```python
from build123d import *

# Parameters (mm, degrees)
EXTRUDE_1_DEPTH        = 3
SHEET_START            = -1
SHEET_METAL_1_DEPTH    = 1
SM_EDGE_FLANGE_1_DEPTH = 60
CUT_EXTRUDE_1_DEPTH    = 149.811702088
CUT_EXTRUDE_2_DEPTH    = 114.368696469
CUT_EXTRUDE_4_DEPTH    = 114.368696469
MIRROR_6_COPY_1_DEPTH  = 149.811702088
SKETCH_13_R            = 5.1
CUT_EXTRUDE_5_DEPTH    = 155.10011472
FILLET_1_R             = 10
CUT_EXTRUDE_6_REACH    = 110.409
SKETCH_15_R            = 2.1


# Read off the part's stored shape, not the designer's step: 轉換-實體1
# Sheet-metal steps are written as plain solids
with BuildPart() as part:
    # Sketch 1 → 填料-伸長1 (new body)
    with BuildSketch(Plane(origin=(0, 0, 0), x_dir=(1, 0, 0), z_dir=(0, 1, 0))):
        Polygon((30, 51.961524227), (-30, 51.961524227), (-60, 0), (-30, -51.961524227), (30, -51.961524227), (60, 0), align=None)
    extrude(amount=EXTRUDE_1_DEPTH)

    # Sheet Metal 1 outline → Sheet Metal 1 (add)
    with BuildSketch(Plane(origin=(0, 0, 0), x_dir=(1, 0, 0), z_dir=(0, 1, 0)).offset(SHEET_START)):
        Polygon((-30, 51.961524227), (-60, 0), (-30, -51.961524227), (30, -51.961524227), (60, 0), (30, 51.961524227), align=None)
    extrude(amount=SHEET_METAL_1_DEPTH)

    # 邊線-凸緣1 section (across the edge) → 邊線-凸緣1 (add)
    with BuildSketch(Plane(origin=(-30, 3, 54.961524227), x_dir=(0, 0, -1), z_dir=(1, 0, 0))):
        with BuildLine():
            Line((-4, 1), (-4, 76))
            Line((-4, 76), (0, 76))
            Line((0, 76), (0, 1))
            ThreePointArc((0, 1), (0.292893219, 0.292893219), (1, 0))
            Line((1, 0), (3, 0))
            Line((3, 0), (3, -4))
            Line((3, -4), (1, -4))
            ThreePointArc((1, -4), (-2.535533906, -2.535533906), (-4, 1))
        make_face()
    sm_edge_flange_1 = extrude(amount=SM_EDGE_FLANGE_1_DEPTH)

    # 草圖9 → 除料-伸長1 (cut, symmetric)
    with BuildSketch(Plane.XY.offset(58.961524227)):
        Polygon((-30, 79), (-30, 14), (-10, 79), align=None)
    cut_extrude_1 = extrude(amount=CUT_EXTRUDE_1_DEPTH, both=True, mode=Mode.SUBTRACT)

    # 草圖10 → 除料-伸長2 (cut, through all)
    with BuildSketch(Plane(origin=(0, 3, 0), x_dir=(1, 0, 0), z_dir=(0, 1, 0))):
        Polygon((10, 17.320508076), (-10, 17.320508076), (-20, 0), (-10, -17.320508076), (10, -17.320508076), (20, 0), align=None)
    extrude(amount=-CUT_EXTRUDE_2_DEPTH, mode=Mode.SUBTRACT)

    # 草圖12 → 除料-伸長4 (cut, symmetric)
    with BuildSketch(Plane(origin=(0, 3, 0), x_dir=(1, 0, 0), z_dir=(0, 1, 0))):
        Polygon((50, 295.043861202), (50, 17.320508076), (50, -17.320508076), (50, -295.043861202), (605.446706252, -295.043861202), (605.446706252, 295.043861202), align=None)
    cut_extrude_4 = extrude(amount=CUT_EXTRUDE_4_DEPTH, both=True, mode=Mode.SUBTRACT)

    # 鏡射1: 除料-伸長1 across plane
    add(cut_extrude_1.mirror(Plane(origin=(0, 0, 0), x_dir=(0, 0, 1), z_dir=(1, 0, 0))), mode=Mode.SUBTRACT)

    # 鏡射6: 邊線-凸緣1, 除料-伸長1 across plane
    add(sm_edge_flange_1.mirror(Plane.XY))
    add(cut_extrude_1.mirror(Plane.XY), mode=Mode.SUBTRACT)

    # 鏡射6 copy 1 sketch → 鏡射6 copy 1 (cut, symmetric)
    with BuildSketch(Plane(origin=(0, 0, -58.961524227), x_dir=(-1, 0, 0), z_dir=(0, 0, -1))):
        Polygon((-30, 79), (-30, 14), (-10, 79), align=None)
    extrude(amount=MIRROR_6_COPY_1_DEPTH, both=True, mode=Mode.SUBTRACT)

    # 草圖13 → 除料-伸長5 (cut, through all)
    with BuildSketch(Plane.XY.offset(58.961524227)):
        with Locations((0, 60)):
            Circle(SKETCH_13_R)
    extrude(amount=-CUT_EXTRUDE_5_DEPTH, mode=Mode.SUBTRACT)

    # 圓角1
    fillet_1_edges = [part.edges().sort_by_distance(p)[0] for p in [
        (10, 79, 56.961524227),
        (10, 79, -56.961524227),
        (-10, 79, -56.961524227),
        (-10, 79, 56.961524227),
    ]]
    fillet(fillet_1_edges, radius=FILLET_1_R)

    # 鏡射7: 除料-伸長4 across plane
    add(cut_extrude_4.mirror(Plane(origin=(0, 0, 0), x_dir=(0, 0, 1), z_dir=(1, 0, 0))), mode=Mode.SUBTRACT)

    # 草圖15 → 除料-伸長6 (cut, up to next)
    with BuildSketch(Plane(origin=(0, 3, 0), x_dir=(1, 0, 0), z_dir=(0, 1, 0)), mode=Mode.PRIVATE) as cut_extrude_6_sk1:
        with Locations(Location((-35, 0, 0), (0, 0, 270))):
            Circle(SKETCH_15_R)
    cut_extrude_6_tool1 = extrude(cut_extrude_6_sk1.sketch, amount=-CUT_EXTRUDE_6_REACH, mode=Mode.PRIVATE) & part.part
    # 草圖15 → 除料-伸長6 (cut, up to next)
    with BuildSketch(Plane(origin=(0, 3, 0), x_dir=(1, 0, 0), z_dir=(0, 1, 0)), mode=Mode.PRIVATE) as cut_extrude_6_sk2:
        with Locations(Location((-25, 35, 0), (0, 0, 270))):
            Circle(SKETCH_15_R)
    cut_extrude_6_tool2 = extrude(cut_extrude_6_sk2.sketch, amount=-CUT_EXTRUDE_6_REACH, mode=Mode.PRIVATE) & part.part
    # 草圖15 → 除料-伸長6 (cut, up to next)
    with BuildSketch(Plane(origin=(0, 3, 0), x_dir=(1, 0, 0), z_dir=(0, 1, 0)), mode=Mode.PRIVATE) as cut_extrude_6_sk3:
        with Locations(Location((25, 35, 0), (0, 0, 270))):
            Circle(SKETCH_15_R)
    cut_extrude_6_tool3 = extrude(cut_extrude_6_sk3.sketch, amount=-CUT_EXTRUDE_6_REACH, mode=Mode.PRIVATE) & part.part
    # 草圖15 → 除料-伸長6 (cut, up to next)
    with BuildSketch(Plane(origin=(0, 3, 0), x_dir=(1, 0, 0), z_dir=(0, 1, 0)), mode=Mode.PRIVATE) as cut_extrude_6_sk4:
        with Locations(Location((25, -35, 0), (0, 0, 270))):
            Circle(SKETCH_15_R)
    cut_extrude_6_tool4 = extrude(cut_extrude_6_sk4.sketch, amount=-CUT_EXTRUDE_6_REACH, mode=Mode.PRIVATE) & part.part
    # 草圖15 → 除料-伸長6 (cut, up to next)
    with BuildSketch(Plane(origin=(0, 3, 0), x_dir=(1, 0, 0), z_dir=(0, 1, 0)), mode=Mode.PRIVATE) as cut_extrude_6_sk5:
        with Locations(Location((-25, -35, 0), (0, 0, 270))):
            Circle(SKETCH_15_R)
    cut_extrude_6_tool5 = extrude(cut_extrude_6_sk5.sketch, amount=-CUT_EXTRUDE_6_REACH, mode=Mode.PRIVATE) & part.part
    # 草圖15 → 除料-伸長6 (cut, up to next)
    with BuildSketch(Plane(origin=(0, 3, 0), x_dir=(1, 0, 0), z_dir=(0, 1, 0)), mode=Mode.PRIVATE) as cut_extrude_6_sk6:
        with Locations(Location((35, 0, 0), (0, 0, 270))):
            Circle(SKETCH_15_R)
    cut_extrude_6_tool6 = extrude(cut_extrude_6_sk6.sketch, amount=-CUT_EXTRUDE_6_REACH, mode=Mode.PRIVATE) & part.part
    add(cut_extrude_6_tool1.solids().sort_by_distance((-35, 3, 0))[0], mode=Mode.SUBTRACT)
    add(cut_extrude_6_tool2.solids().sort_by_distance((-25, 3, -35))[0], mode=Mode.SUBTRACT)
    add(cut_extrude_6_tool3.solids().sort_by_distance((25, 3, -35))[0], mode=Mode.SUBTRACT)
    add(cut_extrude_6_tool4.solids().sort_by_distance((25, 3, 35))[0], mode=Mode.SUBTRACT)
    add(cut_extrude_6_tool5.solids().sort_by_distance((-25, 3, 35))[0], mode=Mode.SUBTRACT)
    add(cut_extrude_6_tool6.solids().sort_by_distance((35, 3, 0))[0], mode=Mode.SUBTRACT)


solid = part.part
```
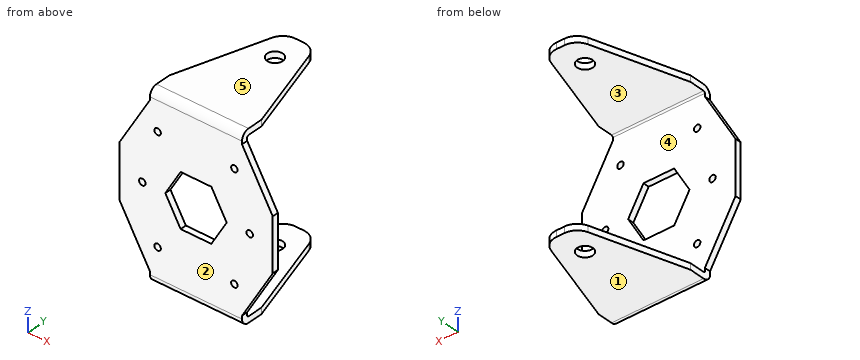
Part model, mm, in its own coordinate system. Face numbers are marked on the shaded views. A direction names the side the tool comes from. Round coordinates to 2 decimals unless told otherwise and drop trailing zeros. Write each loop counter-clockwise with the first axis right and the second up, starting at its lowest first coordinate (ties: lowest second). Pieces come first, ordered by that corner, then holes. Notation, with made-up numbers: M -14,71.25 L 40,71.25 A24 cw 40,85.25 Z; hole C 46,17.5 d2. An arc over 180 degrees is marked long. Answer as CSV lines item,"result". Start each with the question number.
1) Band-saw the part on B-B (y = 47). List the corners of the cut face in (x, z), then the cut area to 3 significant figures.
2) Drill centre lines: L1, parallel to X at y = 1, z = 0; L2, parallel to Z at x = -19.5, y = 38; L3, parallel to Y at x = 22.5, z = 49. Where is each one in solid material? Low to high.
3) Band-saw the part on A-A (x = 25). List the corners of the cut face in (y, z).
4) Which spindle directions (+Z, -Z, +X, -X, +Y, -Y) get a long thin tool onto all of the face, cutting with end or side? Do the marked faces 4 and 5. Say none if no direction does.
5) Band-saw the part on C-C (z = 35). List the corners of the cut face in (x, y), then the cut area to 3 significant figures.
6) Band-saw the part on D-D (x = 14). List the corners of the cut face in (y, z), then the cut area to 3 significant figures.
7) Drop flat-ended pins along their axis: pin 1 (2 mm diameter, centred on x = 4.5, y = 0.5, fed in from +Z); pin 2 (5.5 mm diameter, centred on y = 7, z = 56, fed in from +X); pin 3 (5.5 mm diameter, centred on x = -25, z = 35, fed in from +Y). Give the stop position or say it passes through.
8) Mould opens along Z. For the marked faces 1, 2 and 3 say: +Z half, -Z half, draft (parallel to the pull), parting line (faces both ways), or undercut.
Worked out:
1,outline,"M -19.85,-58.96 L 19.85,-58.96 L 19.85,-54.96 L -19.85,-54.96 Z; M -19.85,54.96 L 19.85,54.96 L 19.85,58.96 L -19.85,58.96 Z"
1,area,"318 mm²"
2,L1,"-50 to -37.1, -32.9 to -20, 20 to 32.9, 37.1 to 50"
2,L2,"-58.96 to -54.96, 54.96 to 58.96"
2,L3,"-1 to 3"
3,outline,"M -1,-53.96 A5 ccw 4,-58.96 L 30.25,-58.96 L 30.25,-54.96 L 4,-54.96 A1 cw 3,-53.96 L 3,-37.1 L -1,-37.1 Z; M -1,-32.9 L 3,-32.9 L 3,32.9 L -1,32.9 Z; M -1,37.1 L 3,37.1 L 3,53.96 A1 cw 4,54.96 L 30.25,54.96 L 30.25,58.96 L 4,58.96 A5 ccw -1,53.96 Z"
4,face 4,"+X, -X, +Y"
4,face 5,"+Z, +X, -X, +Y, -Y"
5,outline,"M -39.79,-1 L -27.1,-1 L -27.1,3 L -39.79,3 Z; M -22.9,-1 L 22.9,-1 L 22.9,3 L -22.9,3 Z; M 27.1,-1 L 39.79,-1 L 39.79,3 L 27.1,3 Z"
5,area,"285 mm²"
6,outline,"M -1,-53.96 A5 ccw 4,-58.96 L 66,-58.96 L 66,-54.96 L 4,-54.96 A1 cw 3,-53.96 L 3,-10.39 L -1,-10.39 Z; M -1,10.39 L 3,10.39 L 3,53.96 A1 cw 4,54.96 L 66,54.96 L 66,58.96 L 4,58.96 A5 ccw -1,53.96 Z"
6,area,"882 mm²"
7,pin 1,"z = 58.29"
7,pin 2,"x = 30"
7,pin 3,"y = 3"
8,face 1,"-Z half"
8,face 2,"draft"
8,face 3,"undercut"
